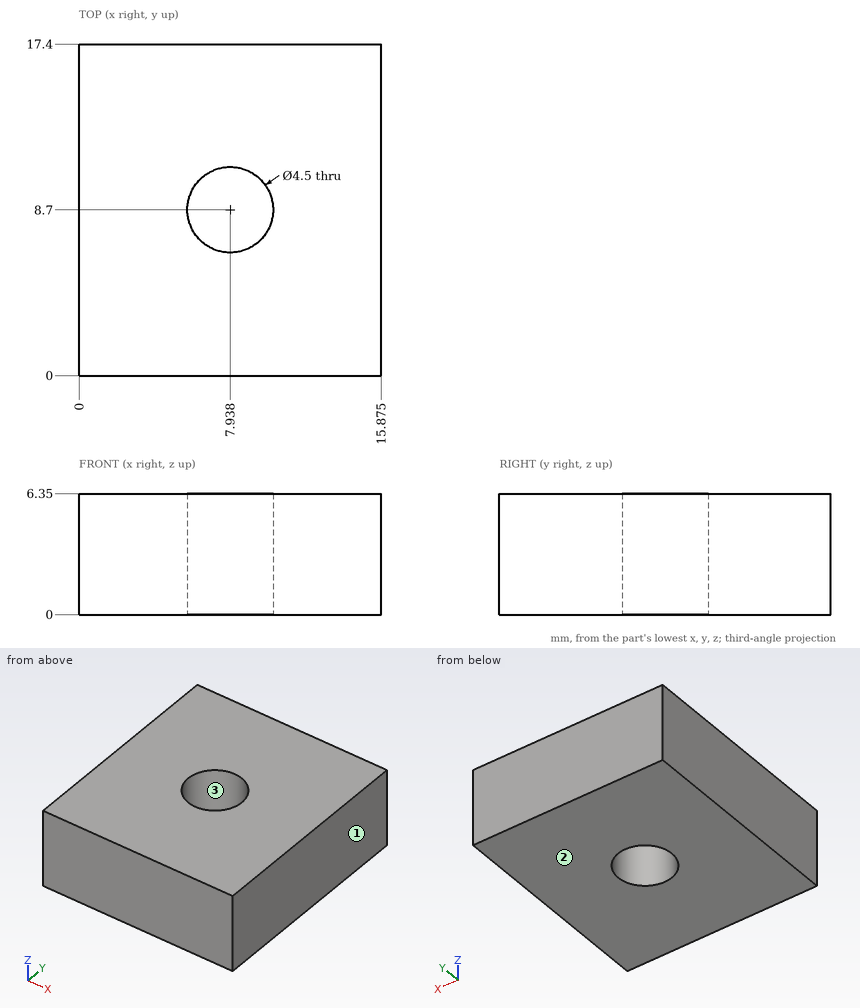
Could you check a few things on this drawing? It's one solid part, dimensions in mm from its lowest x, y, z. Coordinates: 2 decimals unless noted, no trailing zeros. Use a Markdown table: item, result. Add a question column.
Q1. I'm going to push flat-ended pins straight in: pin 1 (5 mm diameter, centred on x = 11, y = 7, fed in from -Z); pin 2 (2.5 mm diameter, centred on x = 7.94, y = 8.7, fed in from -Z). Where does each tip first touch, or does it pass through?
Q2. We'd pull the mould along X, two halves only. Please class the marked faces 1, 2 and 3: pulls with the +X half, pulls with the -X half, needs draft (parallel to the pull), parting line crosses it, or undercut.
Q3. If I drill on L1, parallel to Y at x = 9, z = 4.75 (1 decimal); L2, parallel to X at y = 7.25, z = 2.5 (1 decimal); L3, parallel to X at y = 7.5, z = 3.25 (1 decimal), over which ranges is the centre line in solid material (lowest first)?
Checked values:
| question | item | result |
|---|---|---|
| 1 | pin 1 | z = 0 |
| 1 | pin 2 | through |
| 2 | face 1 | pulls with the +X half |
| 2 | face 2 | needs draft |
| 2 | face 3 | undercut |
| 3 | L1 | 0 to 6.7, 10.7 to 17.4 |
| 3 | L2 | 0 to 6.2, 9.7 to 15.9 |
| 3 | L3 | 0 to 6, 9.8 to 15.9 |
